Autodesk Fusion 360 part; units mm, degrees
sketch "Sketch1" plane through (0, 0, 0) normal (0, 1, 0) x (1, 0, 0)
  line L0 (0, 0) -> (115, 0)
  line L1 (115, -36) -> (0, -36)
  circle A0 centre (5.75, -26) radius 2.15
  circle A1 centre (5.75, -5) radius 2.15
  circle A2 centre (33.75, -5) radius 2.15
  circle A3 centre (33.75, -26) radius 2.15
  circle A4 centre (81.25, -5) radius 2.15
  circle A5 centre (81.25, -26) radius 2.15
  circle A6 centre (109.25, -5.0525) radius 2.15
  circle A7 centre (109.25, -26.0525) radius 2.15
  line L2 (73.45, -36) -> (73.45, 0) construction
  line L3 (41.55, -36) -> (41.55, 0) construction
  line L4 (5.75, -26) -> (39, -26) construction
  line L5 (0, 0) -> (-2.05, 0)
  line L6 (-2.05, 0) -> (-2.05, -36)
  line L7 (-2.05, -36) -> (0, -36)
  line L8 (115, 0) -> (117.05, 0)
  line L9 (117.05, 0) -> (117.05, -36)
  line L10 (117.05, -36) -> (115, -36)
  dimension "d1" = 115
  dimension "d2" = 36
  dimension "d3" = 4.3
  dimension "d4" = 4.3
  dimension "d7" = 21
  dimension "d8" = 5
  dimension "d13" = 4.3
  dimension "d14" = 4.3
  dimension "d15" = 21
  dimension "d16" = 4.3
  dimension "d17" = 4.3
  dimension "d18" = 21
  dimension "d19" = 4.3
  dimension "d20" = 4.3
  dimension "d21" = 21
  dimension "d40" = 28
  dimension "d41" = 28
  dimension "d44" = 28
  dimension "d45" = 28
  dimension "d46" = 5
  dimension "d47" = 7.8
  dimension "d48" = 7.8
  dimension "d50" = 7.8
  dimension "d51" = 7.8
extrude "Extrude1" add sketch "Sketch1" along normal blind 8
sketch "Sketch2" plane through (0, 0, 36) normal (0, 0, 1) x (1, 0, 0)
  line L0 (-2.05, 0) -> (117.05, 0)
  line L1 (117.05, 8) -> (-2.05, 8)
  line L2 (45, 8) -> (70, 8)
  line L3 (70, 8) -> (70, -8)
  line L4 (70, -8) -> (45, -8)
  line L5 (45, -8) -> (45, 8)
  line L6 (45, 8) -> (70, -8) construction
  line L7 (70, 8) -> (45, -8) construction
  circle A0 centre (57.5, -27.1) radius 11
  circle A1 centre (57.5, -27.1) radius 5.4
  circle A2 centre (57.5, -27.1) radius 8
  line L8 (65.5, -27.1) -> (49.5, -27.1) construction
  line L9 (57.5005, -35.1) -> (57.5005, -19.1) construction
  circle A3 centre (65.5, -27.1) radius 2.05
  circle A4 centre (57.5005, -35.1) radius 2.05
  circle A5 centre (49.5, -27.1) radius 2.05
  circle A6 centre (57.5005, -19.1) radius 2.05
  line L10 (70, -8) -> (45, -8)
  line L11 (45, -8) -> (45, -41)
  line L12 (45, -41) -> (70, -41)
  line L13 (70, -41) -> (70, -8)
  line L14 (115, 0) -> (0, 0)
  line L15 (117.05, 0) -> (117.05, 8)
  line L16 (-2.05, 8) -> (-2.05, 0)
  point P0 (57.5, 0)
  dimension "d26" = 25
  dimension "d27" = 16
  dimension "d28" = 22
  dimension "d29" = 10.8
  dimension "d30" = 16
  dimension "d31" = 4.1
  dimension "d32" = 4.1
  dimension "d33" = 4.1
  dimension "d34" = 4.1
  dimension "d35" = 33
  dimension "d39" = 27.1
extrude "Extrude2" add sketch "Sketch2" against normal blind 12 from surface at -14 contours L0 L3 L4 L5 L10 L14 | L4 L10 L11 L12 L13 | A0 | A2 A3 A4 A5 A6
chamfer "Chamfer2" distance 5 angle 45 2 edges at (57.5, 0, 22) (57.5, 0, 10)
extrude "Extrude3" cut sketch "Sketch2" against normal blind 16 contours A0 | A2 A3 A4 A5 A6
extrude "Extrude4" cut sketch "Sketch2" along normal blind 2 from surface at -27 contours A0 | A2 A3 A4 A5 A6
extrude "Extrude5" add 1 faces at (64.771, 8, 18.689) along direction (0, 1, 0) blind 4
sketch "Sketch3" plane through (0, 12, 0) normal (0, 1, 0) x (-1, 0, 0)
  circle A0 centre (-109.25, 5.0525) radius 2.15
  circle A1 centre (-33.75, 26) radius 2.15
  circle A2 centre (-81.25, 26) radius 2.15
  circle A3 centre (-5.75, 5) radius 2.15
  circle A4 centre (-109.25, 26.0525) radius 2.15
  circle A5 centre (-5.75, 26) radius 2.15
  circle A6 centre (-81.25, 5) radius 2.15
  circle A7 centre (-33.75, 5) radius 2.15
  line L0 (-117.05, 0) -> (2.05, 0)
  line L1 (2.05, 0) -> (2.05, 36)
  line L2 (2.05, 36) -> (-117.05, 36)
  line L3 (-117.05, 36) -> (-117.05, 0)
  circle A8 centre (-81.25, 5) radius 4.75
  circle A9 centre (-81.25, 26) radius 4.75
  circle A10 centre (-109.25, 26.0525) radius 4.75
  circle A11 centre (-109.25, 5.0525) radius 4.75
  circle A12 centre (-33.75, 26) radius 4.75
  circle A13 centre (-5.75, 26) radius 4.75
  circle A14 centre (-33.75, 5) radius 4.75
  circle A15 centre (-5.75, 5) radius 4.75
  dimension "d60" = 9.5
  dimension "d61" = 9.5
  dimension "d62" = 9.5
  dimension "d63" = 9.5
  dimension "d64" = 9.5
  dimension "d65" = 9.5
  dimension "d66" = 9.5
  dimension "d67" = 9.5
extrude "Extrude6" add sketch "Sketch3" along normal blind 50 contours L0 L1 L2 L3
extrude "Extrude7" add 1 faces at (37.65, 41.3333, 0) along direction (0, 0, -1) blind 5
chamfer "Chamfer3" distance 5 angle 45 2 edges at (45, 0, 16) (70, 0, 16)
sketch "Sketch4" plane through (0, 0, -5) normal (0, 0, -1) x (-1, 0, 0)
  line L0 (-117.05, 0) -> (2.05, 0)
  line L1 (2.05, 0) -> (2.05, 62)
  line L2 (2.05, 62) -> (-117.05, 62)
  line L3 (-117.05, 62) -> (-117.05, 0)
  line L4 (-77.5, 32) -> (-37.5, 32)
  line L5 (-37.5, 32) -> (-37.5, 28)
  line L6 (-37.5, 28) -> (-77.5, 28)
  line L7 (-77.5, 28) -> (-77.5, 32)
  line L8 (-57.5, 62) -> (-57.5, 32) construction
  line L9 (-57.5, 28) -> (-57.5, 0) construction
  dimension "d73" = 40
  dimension "d74" = 4
  dimension "d75" = 30
  dimension "d78" = 20
extrude "Extrude8" cut sketch "Sketch4" against normal blind 50 contours L4 L5 L6 L7
Can you work these out from the model? Positions are in its coordinate system, mm. A direction names the side the tool comes from. Round coordinates to 2 decimals unless told otherwise and drop trailing zeros. Loops run counter-clockwise (first coordinate to the right, second up) from the corner with the lowest first, then second, coordinate; pieces in that order, holes last. Notation, with made-up numbers: (76.25, -5.5) - (100.25, -5.5) arc R19 ccw to (100.25, 9.5) - close; hole circle Ø7 at (-26.75, -32). An arc over 180 degrees is marked (long way). Write item = value, one per line. Start each with the question number.
(1) If I drill on probe 1 along Z at (x, y) = (85, 53); probe 2 along Z at (x, y) = (109.25, 6.25); probe 3 along X at (y, z) = (2.5, 5), over which ranges is the centre line in solid material (lowest first)? Write a range as [from, to].
(2) If we section it at A-A (y = -27.1): Please give me the cut outline in (x, z), and give its area (3 significant figures).
(3) If we mould it in two halves opening along Z, with no side actions, what happens to faces 1 (the face through (79.544, 5.916, 24.692)), 2 (the face through (77.5, 30, 15)), 3 (the face through (57, -15, 10)), 4 (the face through (36, 12, 6))? For each: released by +Z, released by -Z, zero draft, split by the parting line, or undercut.
(4) If we section it at C-C (x = 57.5): Give the number of separate pieces and of enclosed holes in the cut face, and give its area (3 significant figures).
(5) If we section it at B-B (x = 109.25): Please give me the cut outline in (y, z), and give its area (3 significant figures).
(6) For P1, Ø4, axis at x = 94, z = 3.5, coming from the -Y side; P2, Ø5.5, axis at x = 81.25, z = 26, coming from the +Y side; P3, Ø12, axis at y = -23.5, z = 3.5, coming from the -X side (1 decimal); P4, Ø13, axis at x = 57.5, y = -27.1, coming from the -Z side, each with a flat end and sliding along its axis, tell me the tip position at first contact or that it passes through.
(7) For faces 5 (the face through (70, -23, 16)), 6 (the face through (46.51, -26.62, 21.01)), 7 (the face through (80, 12, 28)), 8 (the face through (57, 28, 15)), which set-ups out of +Z, -Z, +X, -X, +Y, -Y let a thin tool reach every point of the face, with its end or its side?
Ans:
q1.probe_1 = [-5, 2.08], [7.92, 23.08], [28.92, 36]
q1.probe_2 = [-5, 2.9], [7.2, 23.9], [28.2, 36]
q1.probe_3 = [-2.05, 3.6], [7.9, 31.6], [35.9, 79.1], [83.4, 107.1], [111.4, 117.05]
q2.outline = (45, 10) - (46.5, 10) - (46.5, 11) - (47.45, 11) - (47.45, 20) - (46.5, 20) - (46.5, 22) - (45, 22) - close; (51.55, 11) - (52.1, 11) - (52.1, 20) - (51.55, 20) - close; (62.9, 11) - (63.45, 11) - (63.45, 20) - (62.9, 20) - close; (67.55, 11) - (68.5, 11) - (68.5, 10) - (70, 10) - (70, 22) - (68.5, 22) - (68.5, 20) - (67.55, 20) - close
q2.area = 63.0 mm²
q3.face_1 = undercut
q3.face_2 = zero draft
q3.face_3 = released by -Z
q3.face_4 = undercut
q4.separate_pieces = 5
q4.enclosed_holes = 0
q4.area = 2,660 mm²
q5.outline = (0, -5) - (62, -5) - (62, 0.3) - (12, 0.3) - (12, 2.9) - (0, 2.9) - close; (0, 7.2) - (12, 7.2) - (12, 9.8) - (62, 9.8) - (62, 21.3) - (12, 21.3) - (12, 23.9) - (0, 23.9) - close; (0, 28.2) - (12, 28.2) - (12, 30.8) - (62, 30.8) - (62, 36) - (0, 36) - close
q5.area = 1,490 mm²
q6.P1 = 0
q6.P2 = 12
q6.P3 = through
q6.P4 = 11
q7.face_5 = +Z, -Z, +X, -Y
q7.face_6 = +Z
q7.face_7 = +Y
q7.face_8 = +Z, -Z
